from build123d import *

# Parameters (mm, degrees)
SKETCH1_R           = 20
SKETCH1_R_2         = 1.5
BOSS_EXTRUDE1_DEPTH = 2
SKETCH2_R           = 16.405
SKETCH2_R_2         = 12.5
BOSS_EXTRUDE2_DEPTH = 17
SKETCH4_R           = 7.62
CUT_EXTRUDE1_DEPTH  = 17


with BuildPart() as part:
    # Sketch1 → Boss-Extrude1 (new body)
    with BuildSketch(Plane.XY):
        Circle(SKETCH1_R)
        with Locations((0, 10)):
            Circle(SKETCH1_R_2, mode=Mode.SUBTRACT)
        with Locations((10, 0)):
            Circle(SKETCH1_R_2, mode=Mode.SUBTRACT)
        with Locations((0, -10)):
            Circle(SKETCH1_R_2, mode=Mode.SUBTRACT)
        with Locations((-10, 0)):
            Circle(SKETCH1_R_2, mode=Mode.SUBTRACT)
    extrude(amount=BOSS_EXTRUDE1_DEPTH)

    # Sketch2 → Boss-Extrude2 (add)
    with BuildSketch(Plane.XY.offset(2)):
        Circle(SKETCH2_R)
        Circle(SKETCH2_R_2, mode=Mode.SUBTRACT)
    extrude(amount=BOSS_EXTRUDE2_DEPTH)

    # Sketch4 → Cut-Extrude1 (cut)
    with BuildSketch(Plane(origin=(0, 0, 0), x_dir=(-1, 0, 0), z_dir=(0, 0, -1))):
        Circle(SKETCH4_R)
    extrude(amount=-CUT_EXTRUDE1_DEPTH, mode=Mode.SUBTRACT)


solid = part.part
Build history of the part. All positions in model axes, mm. A direction names the side the tool comes from. Coordinates: 2 decimals unless noted, no trailing zeros. Write each loop counter-clockwise with the first axis right and the second up, starting at its lowest first coordinate (ties: lowest second). Pieces come first, ordered by that corner, then holes. Notation, with made-up numbers: (9.25, 31.5) -> (53.25, 31.5) arc R27 ccw to (53.25, 47.5) -> close; hole circle Ø1 at (-17.5, 35). An arc over 180 degrees is marked (long way). Use CSV: the item, a comma, the result in double quotes. Start each with the question number.
Q1. Cut at C-C, the plane y = 1. List the corners of the cut face in (x, z), then the cut area to 3 significant figures.
Q2. Pull direction X, two halves, no side cores. Call faces 3 (the cylindrical face through (-0.325, -11.464, 0.986)), 4 (the flat face through (-3.1, 16.4, 2)), 5 (the cylindrical face through (-0.325, 8.536, 0.986)), 6 (the cylindrical face through (-4.336, -19.524, 0.986)): released by +X, released by -X, zero draft, split by the parting line, or undercut.
Q3. Cut at B-B, the plane y = 10. List the corners of the cut face in (x, z), then the cut area to 3 significant figures.
Q4. Drill centre lines: probe 1 along Y at (x, z) = (0, 0.5); probe 2 along Y at (x, z) = (0, 6) (3 decimals); probe 3 along Z at (x, y) = (-12, -15). Where is each one in solid material? Low to high.
Q5. Cut at D-D, the plane x = 9.5. List the corners of the cut face in (y, z), then the cut area to 3 significant figures.
Q6. Flat gauge pins, fed straight in: pin 1 Ø5 at (x, z) = (-1.5, 16.5) entering from +Y (3 decimals); pin 2 Ø2 at (y, z) = (-10.5, 9) entering from +X; pin 3 Ø5 at (x, y) = (-15.5, -8.5) entering from -Z; pin 4 Ø3 at (x, z) = (12, 16.5) entering from +Y. Where does each tip first touch, or does it go through?
Q7. Cut at A-A, the plane x = 0. List the corners of the cut face in (y, z) (3 decimals).
Q8. 3-axis set-ups, long thin cutter, end or side, ignore diameter. For faces 1 (the flat face through (-6, -5, 2)), 2 (the cylindrical face through (1.65, -7.44, 0.99)): which of +Z, -Z, +X, -X, +Y, -Y reach the whole face in a straight line?
Checked values:
1,outline,"(-19.97, 0) -> (-11.12, 0) -> (-11.12, 2) -> (-12.46, 2) -> (-12.46, 19) -> (-16.37, 19) -> (-16.37, 2) -> (-19.97, 2) -> close; (-8.88, 0) -> (-7.55, 0) -> (-7.55, 2) -> (-8.88, 2) -> close; (7.55, 0) -> (8.88, 0) -> (8.88, 2) -> (7.55, 2) -> close; (11.12, 0) -> (19.97, 0) -> (19.97, 2) -> (16.37, 2) -> (16.37, 19) -> (12.46, 19) -> (12.46, 2) -> (11.12, 2) -> close"
1,area,"174 mm²"
2,face 3,"undercut"
2,face 4,"zero draft"
2,face 5,"undercut"
2,face 6,"split by the parting line"
3,outline,"(-17.32, 0) -> (-1.5, 0) -> (-1.5, 2) -> (-7.5, 2) -> (-7.5, 19) -> (-13, 19) -> (-13, 2) -> (-17.32, 2) -> close; (1.5, 0) -> (17.32, 0) -> (17.32, 2) -> (13, 2) -> (13, 19) -> (7.5, 19) -> (7.5, 2) -> (1.5, 2) -> close"
3,area,"250 mm²"
4,probe 1,"y = -20 to -11.5, -8.5 to -7.62, 7.62 to 8.5, 11.5 to 20"
4,probe 2,"y = -16.405 to -12.5, 12.5 to 16.405"
4,probe 3,"z = 0 to 2"
5,outline,"(-17.6, 0) -> (-1.41, 0) -> (-1.41, 2) -> (-8.12, 2) -> (-8.12, 19) -> (-13.37, 19) -> (-13.37, 2) -> (-17.6, 2) -> close; (1.41, 0) -> (17.6, 0) -> (17.6, 2) -> (13.37, 2) -> (13.37, 19) -> (8.12, 19) -> (8.12, 2) -> (1.41, 2) -> close"
5,area,"243 mm²"
6,pin 1,"stops at y = 16.405"
6,pin 2,"stops at x = 13.37"
6,pin 3,"stops at z = 0"
6,pin 4,"stops at y = 12.6"
7,outline,"(-20, 0) -> (-11.5, 0) -> (-11.5, 2) -> (-12.5, 2) -> (-12.5, 19) -> (-16.405, 19) -> (-16.405, 2) -> (-20, 2) -> close; (-8.5, 0) -> (-7.62, 0) -> (-7.62, 2) -> (-8.5, 2) -> close; (7.62, 0) -> (8.5, 0) -> (8.5, 2) -> (7.62, 2) -> close; (11.5, 0) -> (20, 0) -> (20, 2) -> (16.405, 2) -> (16.405, 19) -> (12.5, 19) -> (12.5, 2) -> (11.5, 2) -> close"
8,face 1,"+Z"
8,face 2,"+Z, -Z"
